CAD build for the part. Positions are in the model's coordinates, mm. Coordinates: 2 decimals unless noted, no trailing zeros. Write each loop counter-clockwise with the first axis right and the second up, starting at its lowest first coordinate (ties: lowest second). Pieces come first, ordered by that corner, then holes. Notation, with made-up numbers: (5, 25) -> (31, 25) arc R12 ccw to (31, 32) -> close; hole circle Ø1 at (41.25, 70). An arc over 180 degrees is marked (long way). Answer as CSV lines item,"result". Start each with the question number.
```python
from build123d import *

# Parameters (mm, degrees)
SKETCH1_R           = 1.6256
BOSS_EXTRUDE1_DEPTH = 3.175


with BuildPart() as part:
    # Sketch1 → Boss-Extrude1 (new body)
    with BuildSketch(Plane(origin=(0, 0, 0), x_dir=(1, 0, 0), z_dir=(0, 1, 0))):
        Polygon((0, 28.575), (0, 44.45), (123.19, 44.45), (123.19, 28.575), (128.27, 28.575), (128.27, 15.875), (123.19, 15.875), (123.19, 0), (0, 0), (0, 15.875), (-5.08, 15.875), (-5.08, 28.575), align=None)
        with Locations(Location((-1.5875, 22.225, 0), (0, 0, 270))):
            Circle(SKETCH1_R, mode=Mode.SUBTRACT)
        with Locations(Location((124.7775, 22.225, 0), (0, 0, 270))):
            Circle(SKETCH1_R, mode=Mode.SUBTRACT)
    extrude(amount=BOSS_EXTRUDE1_DEPTH)


solid = part.part
```
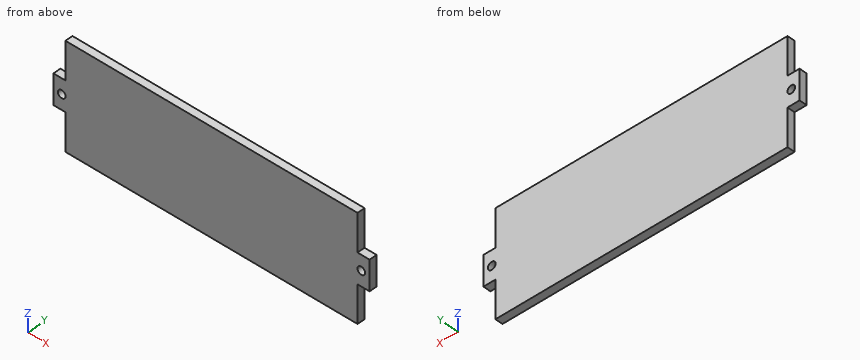
1. Wall check: line 1 (X direction, y = 2.75, z = -34.5). Give the ranges that are in metal, low to high.
2. Flat gauge pins, fed straight in: P1, Ø1.6, axis at x = -1.5, y = 1, coming from the -Z side (3 decimals); P2, Ø2.5, axis at x = -1.59, z = -22.22, coming from the -Y side; P3, Ø1, axis at x = -2, y = 2, coming from the +Z side (3 decimals). Where does each tip first touch, or does it go through?
3. Cut at A-A (y = 0.6). Count the separate pieces of the cut face and the enclosed holes in it, then the cut area to 3 significant figures.
4. Cut at B-B (z = -9). Give the cut face in (x, y) (3 decimals), then the cut area to 3 significant figures.
Geometry check:
1,line 1,"0 to 123.19"
2,P1,"z = -28.575"
2,P2,"through"
2,P3,"z = -15.875"
3,separate pieces,"1"
3,enclosed holes,"2"
3,area,"5,590 mm²"
4,outline,"(0, 0) -> (123.19, 0) -> (123.19, 3.175) -> (0, 3.175) -> close"
4,area,"391 mm²"
